```python
from build123d import *

# Parameters (mm, degrees)
SKETCH_1_W                        = 120
SKETCH_1_H                        = 40
SM_BASE_FLANGE_1_DEPTH            = 4
SM_EDGE_FLANGE_1_STRIP_W          = 17.4732
SM_EDGE_FLANGE_1_STRIP_H          = 4
SM_EDGE_FLANGE_1_STRIP_CUT_DEPTH  = 40
SM_EDGE_FLANGE_1_DEPTH            = 40
SKETCH_12_R                       = 28.5
EXTRUDE_1_DEPTH                   = 4
SKETCH_13_R                       = 6.979767345
CUT_EXTRUDE_2_DEPTH               = 4
SM_EDGE_FLANGE_2_STRIP_W          = 17.4732
SM_EDGE_FLANGE_2_STRIP_H          = 4
SM_EDGE_FLANGE_2_STRIP_CUT_DEPTH  = 40
SM_EDGE_FLANGE_2_RELIEF_W         = 19.4732
SM_EDGE_FLANGE_2_RELIEF_H         = 2
SM_EDGE_FLANGE_2_RELIEF_CUT_DEPTH = 4
SM_EDGE_FLANGE_2_DEPTH            = 40
SKETCH_17_R                       = 28.5
EXTRUDE_2_DEPTH                   = 4


# Sheet-metal steps are written as plain solids
with BuildPart() as part:
    # Sketch 1 → 基体-法兰1 (new body)
    with BuildSketch(Plane.XY):
        Rectangle(SKETCH_1_W, SKETCH_1_H)
    extrude(amount=-SM_BASE_FLANGE_1_DEPTH)

    # 边线-法兰1 strip (across the edge) → 边线-法兰1 strip cut (cut)
    with BuildSketch(Plane(origin=(-60, -20, -4), x_dir=(1, 0, 0), z_dir=(0, 1, 0))):
        with Locations((-4, -2)):
            Rectangle(SM_EDGE_FLANGE_1_STRIP_W, SM_EDGE_FLANGE_1_STRIP_H)
    extrude(amount=SM_EDGE_FLANGE_1_STRIP_CUT_DEPTH, mode=Mode.SUBTRACT)

    # 边线-法兰1 section (across the edge) → 边线-法兰1 (add)
    with BuildSketch(Plane(origin=(-60, -20, -4), x_dir=(1, 0, 0), z_dir=(0, 1, 0))):
        with BuildLine():
            Line((0, 0.7366), (0, 32))
            Line((0, 32), (4, 32))
            Line((4, 32), (4, 0.7366))
            ThreePointArc((4, 0.7366), (4.215745145, 0.215745145), (4.7366, 0))
            Line((4.7366, 0), (4.7366, -4))
            ThreePointArc((4.7366, -4), (1.38731802, -2.61268198), (0, 0.7366))
        make_face()
    extrude(amount=SM_EDGE_FLANGE_1_DEPTH)

    # 草图12 → 凸台-拉伸1 (add)
    with BuildSketch(Plane.ZY.offset(60)):
        with Locations((-40, 0)):
            Circle(SKETCH_12_R)
    extrude(amount=-EXTRUDE_1_DEPTH)

    # 草图13 → 切除-拉伸2 (cut)
    with BuildSketch(Plane.ZY.offset(60)):
        with Locations((-40, 0)):
            Circle(SKETCH_13_R)
    extrude(amount=-CUT_EXTRUDE_2_DEPTH, mode=Mode.SUBTRACT)

    # 边线-法兰2 strip (across the edge) → 边线-法兰2 strip cut (cut)
    with BuildSketch(Plane(origin=(60, -20, -4), x_dir=(0, 1, 0), z_dir=(-1, 0, 0))):
        with Locations((-4, -2)):
            Rectangle(SM_EDGE_FLANGE_2_STRIP_W, SM_EDGE_FLANGE_2_STRIP_H)
    extrude(amount=SM_EDGE_FLANGE_2_STRIP_CUT_DEPTH, mode=Mode.SUBTRACT)

    # 边线-法兰2 relief (on the sheet) → 边线-法兰2 relief cut (cut)
    with BuildSketch(Plane(origin=(60, -15.2634, -4), x_dir=(0, 1, 0), z_dir=(0, 0, -1))):
        with Locations((-7.7366, -41)):
            Rectangle(SM_EDGE_FLANGE_2_RELIEF_W, SM_EDGE_FLANGE_2_RELIEF_H)
    extrude(amount=-SM_EDGE_FLANGE_2_RELIEF_CUT_DEPTH, mode=Mode.SUBTRACT)

    # 边线-法兰2 section (across the edge) → 边线-法兰2 (add)
    with BuildSketch(Plane(origin=(60, -20, -4), x_dir=(0, 1, 0), z_dir=(-1, 0, 0))):
        with BuildLine():
            Line((0, 0.7366), (0, 30))
            Line((0, 30), (4, 30))
            Line((4, 30), (4, 0.7366))
            ThreePointArc((4, 0.7366), (4.215745145, 0.215745145), (4.7366, 0))
            Line((4.7366, 0), (4.7366, -4))
            ThreePointArc((4.7366, -4), (1.38731802, -2.61268198), (0, 0.7366))
        make_face()
    extrude(amount=SM_EDGE_FLANGE_2_DEPTH)

    # 草图17 → 凸台-拉伸2 (add)
    with BuildSketch(Plane.XZ.offset(20)):
        with Locations((40, -40)):
            Circle(SKETCH_17_R)
    extrude(amount=-EXTRUDE_2_DEPTH)


solid = part.part
```
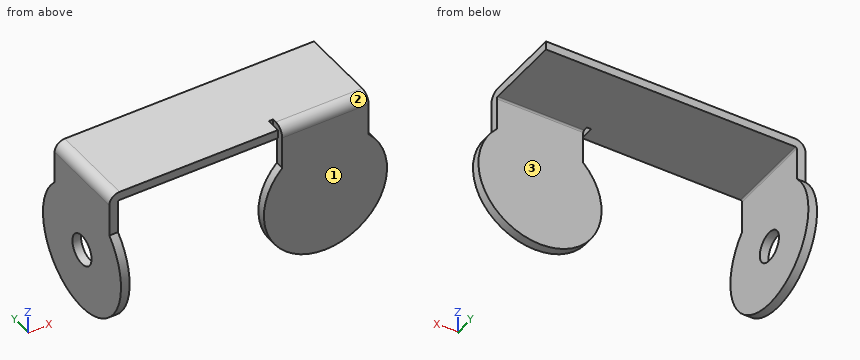
Can you work these out from the model? Positions are in its coordinate system, mm. Face numbers are marked on the shaded views. A direction names the side the tool comes from. Round coordinates to 2 decimals unless told otherwise and drop trailing zeros. Loops run counter-clockwise (first coordinate to the right, second up) from the corner with the lowest first, then second, coordinate; pieces in that order, holes last. Notation, with made-up numbers: (82, -28.75) -> (103, -28.75) arc R12 ccw to (103, -14.75) -> close; hole circle Ø1 at (15.25, 19). An arc over 180 degrees is marked (long way). One line per item, written item: value. Start each with the question number.
1. If we section it at A-A, the plane y = 0: Write out the boundary of the cut face in (x, z).
2. If we section it at C-C, the plane z = -16.5: Write out the boundary of the cut face in (x, y).
3. If I drill on probe 1 along Y at (x, z) = (-57.95, -40); probe 2 along X at (y, z) = (9, -5.5); probe 3 along Z at (x, y) = (25, 15), over which ranges is the centre line in solid material (lowest first)?
4. For pin 1 (11 mm diameter, centred on y = 0, z = -40, fed in from +X); pin 2 (5 mm diameter, centred on y = -19.5, z = -21.5, fed in from +X); pin 3 (3 mm diameter, centred on x = 43, z = -21.5, fed in from -Y); pin 4 (21.5 mm diameter, centred on x = 24.5, z = -9, fed in from +Y), each with a flat end and sliding along its axis, tell me the tip position at first contact or that it passes through.
5. If we section it at D-D, the plane x = 40: Write out the boundary of the cut face in (y, z).
6. For the marked faces 1, 2 and 3, which set-ups out of +Z, -Z, +X, -X, +Y, -Y let a thin tool reach every point of the face, with its end or its side?
7. If we section it at B-B, the plane z = -40: Write out the boundary of the cut face in (x, y).
Calculated:
1. outline: (-60, -68.5) -> (-56, -68.5) -> (-56, -46.98) -> (-60, -46.98) -> close; (-60, -33.02) -> (-56, -33.02) -> (-56, -4.74) arc R0.74 cw to (-55.26, -4) -> (60, -4) -> (60, 0) -> (-55.26, 0) arc R4.74 ccw to (-60, -4.74) -> close
2. outline: (-60, -20) -> (-56, -20) -> (-56, 20) -> (-60, 20) -> close; (20, -20) -> (60, -20) -> (60, -16) -> (20, -16) -> close
3. probe 1: y = -28.5 to -6.98, 6.98 to 28.5
3. probe 2: x = -60 to -56
3. probe 3: z = -4 to 0
4. pin 1: passes through
4. pin 2: stops at x = 63.58
4. pin 3: stops at y = -20
4. pin 4: stops at y = 20
5. outline: (-20, -68.5) -> (-16, -68.5) -> (-16, -4.74) arc R0.74 cw to (-15.26, -4) -> (20, -4) -> (20, 0) -> (-15.26, 0) arc R4.74 ccw to (-20, -4.74) -> close
6. face 1: +Z, -Z, +X, -Y
6. face 2: +Z, +X, -Y
6. face 3: -Z, +X, +Y
7. outline: (-60, -28.5) -> (-56, -28.5) -> (-56, -6.98) -> (-60, -6.98) -> close; (-60, 6.98) -> (-56, 6.98) -> (-56, 28.5) -> (-60, 28.5) -> close; (11.5, -20) -> (68.5, -20) -> (68.5, -16) -> (11.5, -16) -> close
